The figure shows three views and two pictorial views of one solid part (mm, origin at its lowest corner). Answer the questions. A direction names the side the tool comes from. Give positions to 0.01 mm unless a question says otherwise; leave off trailing zeros. Order: outer loops, then holes, each group sorted by start corner. A loop starts at its lowest first (then second) coordinate and runs counter-clockwise, first axis right, second up. Notation, with made-up numbers: (46.25, 85) - (89.25, 85) arc R15 ccw to (89.25, 90) - close; hole circle Ø3 at (2.25, -3.5). An arc over 180 degrees is marked (long way). Use a Markdown table: item, result. Add a question column.
1. A cutting plane is placed at A-A on z = 4.5. Determine the outline of the cut face in (x, y).
2. A cutting plane is placed at D-D on x = 7.25. Determine the outline of the cut face in (y, z), and give its area (3 significant figures).
3. Which of the six approach directions +Z, -Z, +X, -X, +Y, -Y give full straight-line access (tool end or side, diameter ignored) to the marked faces 4, 5 and 6?
4. For a pull along Z with two mould halves and no side action, classify the marked faces 1, 2 and 3 as released by +Z, released by -Z, zero draft, split by the parting line, or undercut.
5. Consider L1, parallel to Z at x = 4.5, y = 2.4; L2, parallel to Z at x = 4.5, y = 0.95. Determine where each line is inside the solid, lowest interval first.
6. Flat-ended cylindrical pins translate along their axes: P1, Ø1, axis at x = 4.5, z = 4.5, coming from the +Y side; P2, Ø1, axis at y = 0.5, z = 6, coming from the +X side; P3, Ø1.5, axis at x = 1.5, y = 2, coming from the -Z side. Find the tip coordinate at first contact, or state that the pin passes through.
7. A cutting plane is placed at C-C on y = 2.1. Determine the outline of the cut face in (x, z), and give its area (3 significant figures).
8. A cutting plane is placed at B-B on x = 4.5. Determine the outline of the cut face in (y, z).
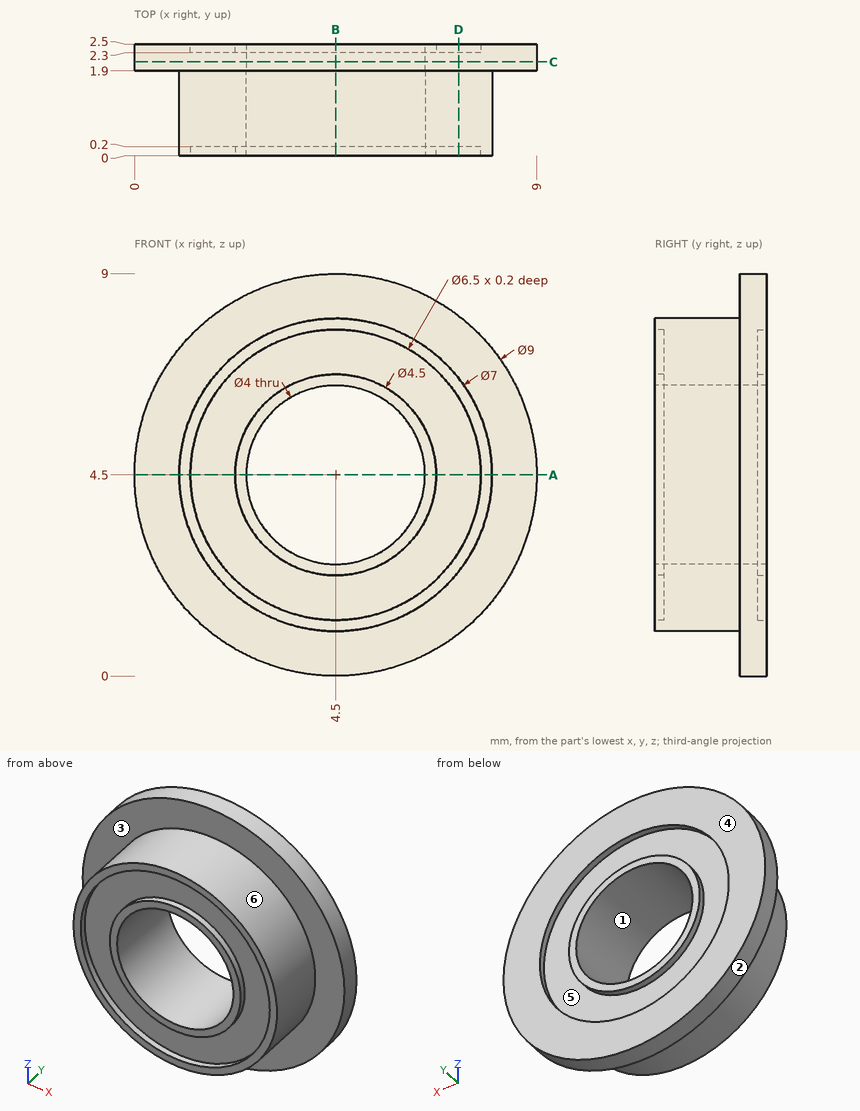
Output values:
| question | item | result |
|---|---|---|
| 1 | outline | (0, 1.9) - (1, 1.9) - (1, 0) - (1.25, 0) - (1.25, 0.2) - (2.25, 0.2) - (2.25, 0) - (2.5, 0) - (2.5, 2.5) - (2.25, 2.5) - (2.25, 2.3) - (1.25, 2.3) - (1.25, 2.5) - (0, 2.5) - close; (6.5, 0) - (6.75, 0) - (6.75, 0.2) - (7.75, 0.2) - (7.75, 0) - (8, 0) - (8, 1.9) - (9, 1.9) - (9, 2.5) - (7.75, 2.5) - (7.75, 2.3) - (6.75, 2.3) - (6.75, 2.5) - (6.5, 2.5) - close |
| 2 | outline | (0, 2.33) - (1.9, 2.33) - (1.9, 0.94) - (2.5, 0.94) - (2.5, 2.77) - (2.3, 2.77) - (2.3, 6.23) - (2.5, 6.23) - (2.5, 8.06) - (1.9, 8.06) - (1.9, 6.67) - (0, 6.67) - (0, 6.23) - (0.2, 6.23) - (0.2, 2.77) - (0, 2.77) - close |
| 2 | area | 11.1 mm² |
| 3 | face 4 | +Z, -Z, +X, -X, +Y |
| 3 | face 5 | +Y |
| 3 | face 6 | -Y |
| 4 | face 1 | undercut |
| 4 | face 2 | split by the parting line |
| 4 | face 3 | zero draft |
| 5 | L1 | 0 to 1.25, 2.25 to 2.5, 6.5 to 6.75, 7.75 to 9 |
| 5 | L2 | 1 to 2.5, 6.5 to 8 |
| 6 | P1 | through |
| 6 | P2 | x = 7.85 |
| 6 | P3 | z = 0.6 |
| 7 | outline | circle Ø9 at (4.5, 4.5); hole circle Ø4 at (4.5, 4.5) |
| 7 | area | 51.1 mm² |
| 8 | outline | (0, 1) - (1.9, 1) - (1.9, 0) - (2.5, 0) - (2.5, 1.25) - (2.3, 1.25) - (2.3, 2.25) - (2.5, 2.25) - (2.5, 2.5) - (0, 2.5) - (0, 2.25) - (0.2, 2.25) - (0.2, 1.25) - (0, 1.25) - close; (0, 6.5) - (2.5, 6.5) - (2.5, 6.75) - (2.3, 6.75) - (2.3, 7.75) - (2.5, 7.75) - (2.5, 9) - (1.9, 9) - (1.9, 8) - (0, 8) - (0, 7.75) - (0.2, 7.75) - (0.2, 6.75) - (0, 6.75) - close |
